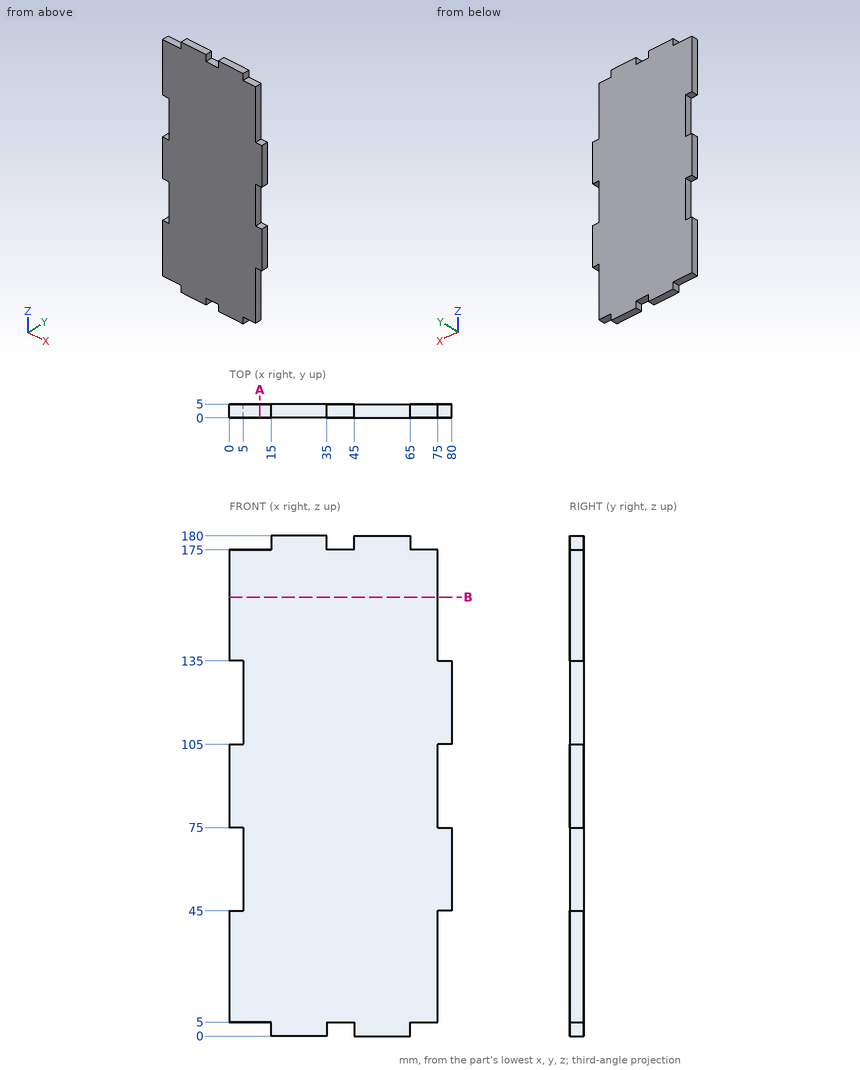
Can you work these out from the drawing? Everything is in mm from the part's minimum corner. Coordinates: 2 decimals unless noted, no trailing zeros. Loops run counter-clockwise (first coordinate to the right, second up) from the corner with the lowest first, then second, coordinate; pieces in that order, holes last.
1) I need wall thicknesses on probe 1 along X at (y, z) = (1.3, 59); probe 2 along X at (y, z) = (4.4, 153); probe 3 along Z at (x, y) = (14.5, 4.85). Which ranges of each line are inside material? Lowest first, please.
2) For pin 1 (1.5 mm diameter, centred on x = 1.5, y = 1.5, fed in from -Z); pin 2 (2.5 mm diameter, centred on y = 3.5, z = 85.5, fed in from +X); pin 3 (2.5 mm diameter, centred on y = 2, z = 178, fed in from -X), each with a flat end and sliding along its axis, tell me the tip position at first contact or that it passes through.
3) Imagine slicing it at B-B on z = 158. List the corners of the cut face in (x, y) for me, plus the area to 3 significant figures.
4) Imagine slicing it at A-A on x = 11. List the corners of the cut face in (y, z) for me, plus the area to 3 significant figures.
Completed:
1. probe 1: x = 5 to 80
1. probe 2: x = 0 to 75
1. probe 3: z = 5 to 175
2. pin 1: stops at z = 5
2. pin 2: stops at x = 75
2. pin 3: stops at x = 15
3. outline: (0, 0) - (75, 0) - (75, 5) - (0, 5) - close
3. area: 375 mm2
4. outline: (0, 5) - (5, 5) - (5, 175) - (0, 175) - close
4. area: 850 mm2
